from build123d import *

# Parameters (mm, degrees)
BOSS_EXTRUDE1_DEPTH       = 15.24
BOSS_EXTRUDE1_DEPTH_BACK  = 76.2
BOSS_EXTRUDE2_DEPTH       = 11.43
SHELL3_T                  = -6.35
BOSS_EXTRUDE9_REACH       = 580.52
BOSS_EXTRUDE4_DEPTH       = 7.62
SHELL4_T                  = -6.35
BOSS_EXTRUDE10_START      = -5.936799282
BOSS_EXTRUDE10_DEPTH      = 5.936799282
BOSS_EXTRUDE11_DEPTH      = 25.4
BOSS_EXTRUDE11_DEPTH_BACK = 25.4
BOSS_EXTRUDE12_REACH      = 744.722


with BuildPart() as part:
    # Sketch3 → Boss-Extrude1 (new, two sides: drawn at the far end of the back side and taken through both)
    with BuildSketch(Plane(origin=(0, 0, 0), x_dir=(1, 0, 0), z_dir=(0, 1, 0)).offset(-BOSS_EXTRUDE1_DEPTH_BACK)):
        with BuildLine():
            Line((-475.154754325, -2.10083146), (-501.46472086, -4.34467525))
            Line((-501.46472086, -4.34467525), (-530.970406525, -16.925757689))
            Line((-530.970406525, -16.925757689), (-541.959235577, -112.906916108))
            ThreePointArc((-541.959235577, -112.906916108), (-423.220596764, -47.00180275), (-325.667958287, -141.478419116))
            Line((-325.667958287, -141.478419116), (-333.580935141, -74.592900266))
            Line((-333.580935141, -74.592900266), (-363.451088866, -24.174556876))
            Line((-363.451088866, -24.174556876), (-449.754754325, -2.10083146))
            ThreePointArc((-449.754754325, -2.10083146), (-462.454754325, -14.800833325), (-475.154754325, -2.10083146))
        make_face()
    extrude(amount=BOSS_EXTRUDE1_DEPTH + BOSS_EXTRUDE1_DEPTH_BACK)

    # Boss-Extrude9: up to this face of the body (flat: up to its plane)
    boss_extrude9_end = Plane(part.part.faces().sort_by_distance((-443.624527124, 15.24, 42.595574003))[0])
    # Sketch11 → Boss-Extrude9 (add, up to the picked face)
    with BuildSketch(Plane(origin=(0, 68.54, 0), x_dir=(1, 0, 0), z_dir=(0, 1, 0)), mode=Mode.PRIVATE) as boss_extrude9_sk1:
        with BuildLine():
            Line((-505.199519379, -28.941561379), (-510.924193781, -42.454904444))
            Line((-510.924193781, -42.454904444), (-468.930038741, -42.454904444))
            ThreePointArc((-468.930038741, -42.454904444), (-474.068166901, -36.548395666), (-475.918740123, -28.941649602))
            Line((-475.918740123, -28.941649602), (-505.199519379, -28.941561379))
        make_face()
    boss_extrude9_tool1 = split(extrude(boss_extrude9_sk1.sketch, amount=-BOSS_EXTRUDE9_REACH, mode=Mode.PRIVATE), bisect_by=boss_extrude9_end, keep=Keep.BOTH, mode=Mode.PRIVATE)


with BuildPart() as body_2:
    # Sketch4 → Boss-Extrude2 (new body)
    with BuildSketch(Plane(origin=(0, 68.54, 0), x_dir=(1, 0, 0), z_dir=(0, 1, 0))):
        with BuildLine():
            Line((-505.199519379, -28.941561379), (-510.924193781, -42.454904444))
            Line((-510.924193781, -42.454904444), (-446.727083924, -108.742597242))
            Line((-446.727083924, -108.742597242), (-432.506297568, -99.706904201))
            Line((-432.506297568, -99.706904201), (-453.485090126, -44.423263798))
            ThreePointArc((-453.485090126, -44.423263798), (-468.76509838, -42.570216845), (-475.918740123, -28.941649602))
            Line((-475.918740123, -28.941649602), (-505.199519379, -28.941561379))
        make_face()
    extrude(amount=-BOSS_EXTRUDE2_DEPTH)

    # Shell3
    shell3_openings = [body_2.faces().sort_by_distance(p)[0] for p in [
        (-469.398872601, 57.11, 63.557756805),
        (-469.398872601, 68.54, 63.557756805),
    ]]
    offset(amount=SHELL3_T, openings=shell3_openings, kind=Kind.INTERSECTION)


with BuildPart() as part_1:
    add(part.part)

    add(body_2.part)  # Boss-Extrude9 merges body 2
    add(boss_extrude9_tool1.solids().sort_by(Axis((-490.927934, 68.54, 36.102447), (0, -1, 0)))[0])

    # Sketch8 → Boss-Extrude10 (add)
    with BuildSketch(Plane(origin=(0, 15.24, 0), x_dir=(1, 0, 0), z_dir=(0, 1, 0)).offset(BOSS_EXTRUDE10_START)):
        with BuildLine():
            Line((-371.049471839, -131.701729119), (-325.667958287, -141.478419116))
            ThreePointArc((-325.667958287, -141.478419116), (-423.220596764, -47.00180275), (-541.959235577, -112.906916108))
            Line((-541.959235577, -112.906916108), (-491.729175354, -110.68768413))
            ThreePointArc((-491.729175354, -110.68768413), (-425.655830818, -88.268337191), (-371.049471839, -131.701729119))
        make_face()
    extrude(amount=BOSS_EXTRUDE10_DEPTH)

    # Sketch9 → Boss-Extrude11 (add, two sides: drawn at the far end of the back side and taken through both)
    with BuildSketch(Plane(origin=(0, 0, 0), x_dir=(1, 0, 0), z_dir=(0, 1, 0)).offset(-BOSS_EXTRUDE11_DEPTH_BACK)):
        with BuildLine():
            Line((-676.938792406, 25.463963625), (-681.369396203, 13.561873472))
            ThreePointArc((-681.369396203, 13.561873472), (-697.932826151, 5.412719448), (-688.863344118, -10.665228762))
            Line((-688.863344118, -10.665228762), (-526.489446237, -51.02276527))
            Line((-526.489446237, -51.02276527), (-525.298257919, -40.618414259))
            Line((-525.298257919, -40.618414259), (-513.502810151, -43.550136784))
            Line((-513.502810151, -43.550136784), (-516.15079803, -66.678801621))
            Line((-516.15079803, -66.678801621), (-691.926688237, -22.990240843))
            ThreePointArc((-691.926688237, -22.990240843), (-710.065652303, 9.165655576), (-676.938792406, 25.463963625))
        make_face()
    extrude(amount=BOSS_EXTRUDE11_DEPTH + BOSS_EXTRUDE11_DEPTH_BACK)

    # Boss-Extrude12: up to this face of the body (flat: up to its plane)
    boss_extrude12_end = Plane(part_1.part.faces().sort_by_distance((-443.624527124, -76.2, 42.595574003))[0])
    # Sketch12 → Boss-Extrude12 (add, up to the picked face)
    with BuildSketch(Plane.XZ.offset(92.130800062), mode=Mode.PRIVATE) as boss_extrude12_sk1:
        with BuildLine():
            Line((-493.29786016, 29.59254273), (-477.784324755, 30.750375257))
            ThreePointArc((-477.784324755, 30.750375257), (-476.661333768, 35.528904506), (-474.321994889, 39.844335441))
            Line((-474.321994889, 39.844335441), (-479.53607938, 43.470681078))
            Line((-479.53607938, 43.470681078), (-495.321687866, 42.29254273))
            Line((-495.321687866, 42.29254273), (-493.29786016, 29.59254273))
        make_face()
    boss_extrude12_tool1 = split(extrude(boss_extrude12_sk1.sketch, amount=-BOSS_EXTRUDE12_REACH, mode=Mode.PRIVATE), bisect_by=boss_extrude12_end, keep=Keep.BOTH, mode=Mode.PRIVATE)


with BuildPart() as body_2_2:
    # Sketch6 → Boss-Extrude4 (new body)
    with BuildSketch(Plane.XZ.offset(92.130800062)):
        with BuildLine():
            Line((-493.29786016, 29.59254273), (-501.65329384, 82.024875489))
            Line((-501.65329384, 82.024875489), (-460.055244029, 108.470724329))
            Line((-460.055244029, 108.470724329), (-436.590495923, 84.974770196))
            Line((-436.590495923, 84.974770196), (-454.490501674, 46.803141976))
            ThreePointArc((-454.490501674, 46.803141976), (-469.864919046, 44.185661822), (-477.784324755, 30.750375257))
            Line((-477.784324755, 30.750375257), (-493.29786016, 29.59254273))
        make_face()
    extrude(amount=-BOSS_EXTRUDE4_DEPTH)

    # Shell4
    shell4_openings = [body_2_2.faces().sort_by_distance(p)[0] for p in [
        (-471.64936301, -84.510800062, 70.060968027),
        (-471.64936301, -92.130800062, 70.060968027),
    ]]
    offset(amount=SHELL4_T, openings=shell4_openings, kind=Kind.INTERSECTION)


with BuildPart() as part_2:
    add(part_1.part)

    add(body_2_2.part)  # Boss-Extrude12 merges body 2 2
    add(boss_extrude12_tool1.solids().sort_by(Axis((-485.45228, -92.1308, 36.761722), (0, 1, 0)))[0])


solid = part_2.part
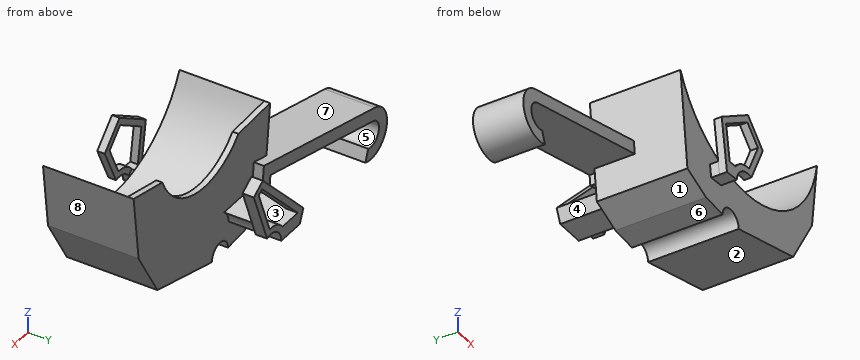
Here's how the part is built. I have some questions about the finished solid (model axes, mm). Face numbers are marked on the shaded views. A direction names the side the tool comes from. Give positions to 0.01 mm unless a question says otherwise; leave off trailing zeros. Loops run counter-clockwise (first coordinate to the right, second up) from the corner with the lowest first, then second, coordinate; pieces in that order, holes last. Notation, with made-up numbers: (-33.5, 1) -> (-17.5, 1) arc R34 cw to (-17.5, 35) -> close; hole circle Ø3 at (39.5, -34). An arc over 180 degrees is marked (long way). One line per item, written item: value.
Q1. If I drill on line 1 along Y through (x, z) = (-584.5, 46.5); line 2 along X through (y, z) = (10, 97.5); line 3 along X through (y, z) = (-6.5, 96.5), over which ranges is the centre line in solid material (lowest first)?
Answers follow:
line 1: -25.4 to 25.4
line 2: -540.2 to -475.51, -400.79 to -330.87
line 3: -540.08 to -532.81, -343.49 to -330.99
Q2. We'd pull the mould along X, two halves only. Please class the marked faces 6, 7 and 8: pulls with the +X half, pulls with the -X half, needs draft (parallel to the pull), parting line crosses it, or undercut.
Answers follow:
face 6: undercut
face 7: pulls with the -X half
face 8: pulls with the +X half
Q3. Suppose I cut it at A-A on y = -67. Please give me the cut outline in (x, z), then the cut area to 3 significant figures.
Answers follow:
outline: (-541.96, 112.91) -> (-530.97, 16.93) -> (-501.46, 4.34) -> (-475.15, 2.1) arc R12.7 cw to (-449.75, 2.1) -> (-363.45, 24.17) -> (-333.58, 74.59) -> (-325.67, 141.48) arc R114 cw to start
area: 9,660 mm^2
Q4. On a 3-axis mill with a long thin cutter (end or side, diameter ignored), from which of +Z, -Z, +X, -X, +Y, -Y can I reach the whole of each face in a straight line? I mean the marked faces 1, 2, 3, 4 and 5. Say none if no direction works.
Answers follow:
face 1: -Z, +Y, -Y
face 2: -Z, +X, +Y, -Y
face 3: none
face 4: -Z, +Y
face 5: +Y, -Y
Q5. I'm going to push flat-ended pins straight in: pin 1 Ø10 at (x, y) = (-513, -47.5) entering from -Z; pin 2 Ø12.5 at (x, y) = (-492.5, 28.5) entering from +Z; pin 3 Ø3 at (y, z) = (-49.5, 8) entering from -X. Where does each tip first touch, or does it pass through?
Answers follow:
pin 1: z = 7.13
pin 2: z = 42.45
pin 3: x = -513.56
Q6. Suppose I cut it at C-C on y = -17. Please give me the cut outline in (x, z), then the cut area to 3 significant figures.
Answers follow:
outline: (-691.93, 22.99) arc R25.4 ccw (long way) to (-676.94, -25.46) -> (-681.37, -13.56) arc R12.7 cw (long way) to (-688.86, 10.67) -> (-534.64, 49) -> (-530.97, 16.93) -> (-501.46, 4.34) -> (-475.15, 2.1) arc R12.7 cw to (-449.75, 2.1) -> (-363.45, 24.17) -> (-333.58, 74.59) -> (-325.67, 141.48) arc R114 cw to (-541.96, 112.91) -> (-536.1, 61.72) -> close
area: 12,500 mm^2
Q7. Suppose I cut it at B-B on x = -591.5. Please give me the cut outline in (y, z), then the cut area to 3 significant figures.
Answers follow:
outline: (-25.4, 34.86) -> (25.4, 34.86) -> (25.4, 47.95) -> (-25.4, 47.95) -> close
area: 665 mm^2
